Check sheet for the drawn part. Datum: minimum x, y, z corner. Units: mm. Coordinates: 2 decimals unless noted, no trailing zeros. Order: outer loops, then holes, each group sorted by start corner. A loop starts at its lowest first (then second) coordinate and runs counter-clockwise, first axis right, second up.
1. Cross-section at B-B (x = 88.9). Enter the section's corners in (y, z), then the cut area to 3 significant figures.
2. Cross-section at C-C (z = 2). Enter the section's corners in (x, y), then the cut area to 3 significant figures.
3. Cross-section at A-A (y = 88.9). Enter the section's corners in (x, z).
4. Gauge pin test, flat ends, axial feed: pin 1 Ø2 at (x, y) = (113.5, 119.5) entering from -Z; pin 2 Ø4 at (x, y) = (38, 32.5) entering from +Z. Record the tip position at first contact, or that the pin passes through.
5. Thickness scan on line 1 (Y direction, x = 88.9, z = 2.8); line 2 (Z direction, x = 141, y = 55.5); line 3 (Y direction, x = 122, z = 1). Record the ranges inside material, lowest first.
6. Cross-section at D-D (y = 12.7). Enter the section's corners in (x, z).
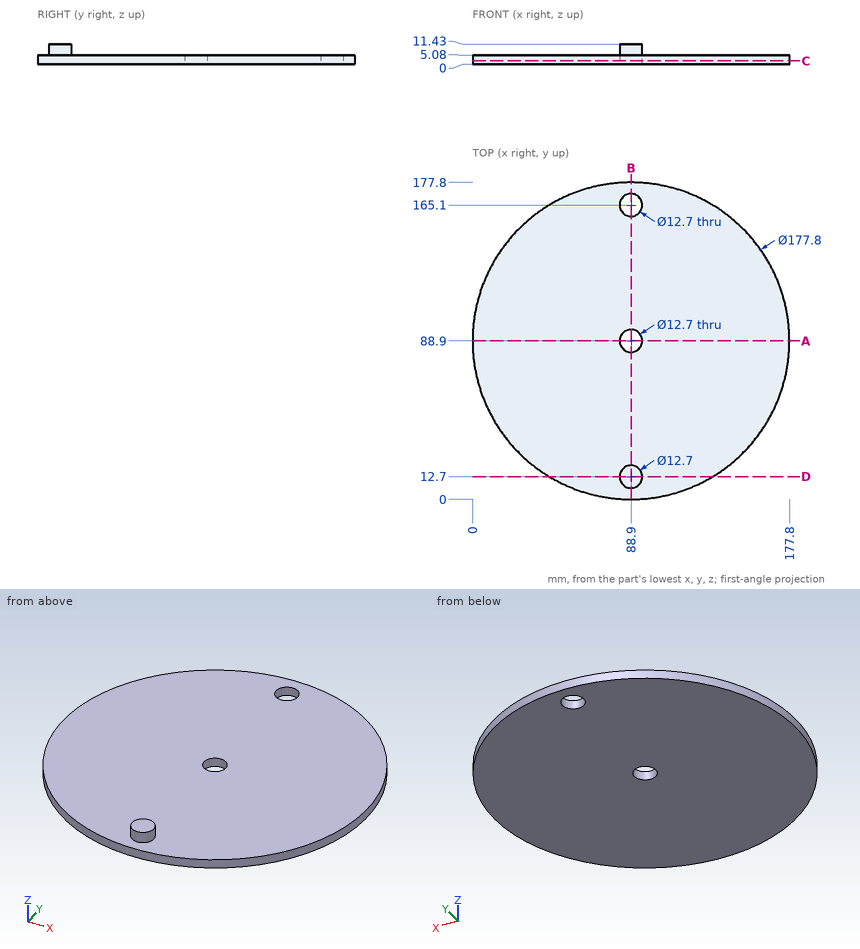
Data:
1. outline: (0, 0) - (82.55, 0) - (82.55, 5.08) - (19.05, 5.08) - (19.05, 11.43) - (6.35, 11.43) - (6.35, 5.08) - (0, 5.08) - close; (95.25, 0) - (158.75, 0) - (158.75, 5.08) - (95.25, 5.08) - close; (171.45, 0) - (177.8, 0) - (177.8, 5.08) - (171.45, 5.08) - close
1. area: 855 mm2
2. outline: circle Ø177.8 at (88.9, 88.9); hole circle Ø12.7 at (88.9, 88.9); hole circle Ø12.7 at (88.9, 165.1)
2. area: 24,600 mm2
3. outline: (0, 0) - (82.55, 0) - (82.55, 5.08) - (0, 5.08) - close; (95.25, 0) - (177.8, 0) - (177.8, 5.08) - (95.25, 5.08) - close
4. pin 1: stops at z = 0
4. pin 2: stops at z = 5.08
5. line 1: y = 0 to 82.55, 95.25 to 158.75, 171.45 to 177.8
5. line 2: z = 0 to 5.08
5. line 3: y = 6.39 to 171.41
6. outline: (43.11, 0) - (134.69, 0) - (134.69, 5.08) - (95.25, 5.08) - (95.25, 11.43) - (82.55, 11.43) - (82.55, 5.08) - (43.11, 5.08) - close
